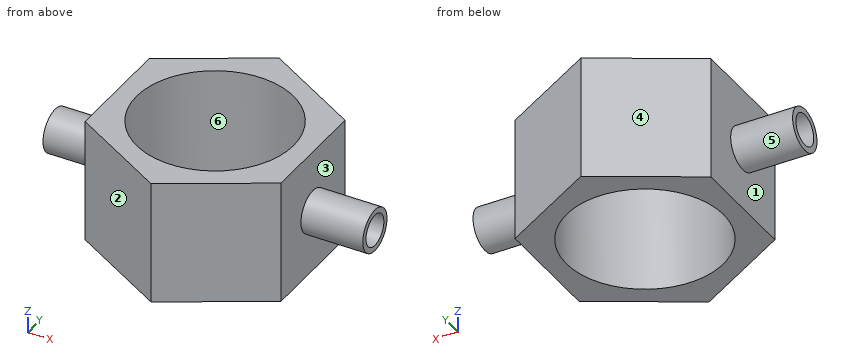
```python
from build123d import *

# Parameters (mm, degrees)
F1_DEPTH  = 12.7
F2_R      = 16.11687381
F3_DEPTH  = 25.4
F4_R      = 4.4261898193
F5_DEPTH  = 12.7
F6_R      = 4.3771900823
F7_DEPTH  = 12.7
F8_R      = 3.2385
F9_DEPTH  = 7.62
F10_R     = 3.2422174322
F11_DEPTH = 7.62


with BuildPart() as f1:
    # F0 (on Top) → F1 (new body, symmetric)
    with BuildSketch(Plane.XY):
        Polygon((-20.0972985476, -2.401636506), (-20.0972985476, -25.6079979589), (0, -37.2111786854), (20.0972985476, -25.6079979589), (20.0972985476, -2.401636506), (0, 9.2015442204), align=None)
    extrude(amount=F1_DEPTH, both=True)

    # F2 (on face) → F3 (cut)
    with BuildSketch(Plane.XY.offset(12.7)):
        with Locations((0, -14.0048172325)):
            Circle(F2_R)
    extrude(amount=-F3_DEPTH, mode=Mode.SUBTRACT)

    # F4 (on face) → F5 (join)
    with BuildSketch(Plane(origin=(-20.0972985476, 0, 0), x_dir=(0, -1, 0), z_dir=(-1, 0, 0))):
        with Locations((14.0048172325, 0)):
            Circle(F4_R)
    extrude(amount=F5_DEPTH)

    # F6 (on face) → F7 (join)
    with BuildSketch(Plane.YZ.offset(20.0972985476)):
        with Locations((-14.0048172325, 0)):
            Circle(F6_R)
    extrude(amount=F7_DEPTH)

    # F8 (on face) → F9 (cut)
    with BuildSketch(Plane(origin=(-32.7972985476, 0, 0), x_dir=(0, -1, 0), z_dir=(-1, 0, 0))):
        with Locations((14.0048172325, 0)):
            Circle(F8_R)
    extrude(amount=-F9_DEPTH, mode=Mode.SUBTRACT)

    # F10 (on face) → F11 (cut)
    with BuildSketch(Plane.YZ.offset(32.7972985476)):
        with Locations((-14.0048172325, 0)):
            Circle(F10_R)
    extrude(amount=-F11_DEPTH, mode=Mode.SUBTRACT)


solid = f1.part
```
Read the model definition and answer for the solid it produces. Units are mm, in the model's axes. Face numbers are marked on the shaded views. A direction names the side the tool comes from. Round coordinates to 2 decimals unless told otherwise and drop trailing zeros. Write each loop counter-clockwise with the first axis right and the second up, starting at its lowest first coordinate (ties: lowest second). Pieces come first, ordered by that corner, then holes. Notation, with made-up numbers: (9.25, -14) - (23.25, -14) arc R18 cw to (23.25, -7) - close; hole circle Ø1 at (-39.75, 88). An arc over 180 degrees is marked (long way). Use CSV: the item, a comma, the result in double quotes.
Q1. Find section A-A, the plane y = -5. Write down the section's boundary in (x, z).
Values:
outline,"(-20.1, -12.7) - (-13.37, -12.7) - (-13.37, 12.7) - (-20.1, 12.7) - close; (13.37, -12.7) - (20.1, -12.7) - (20.1, 12.7) - (13.37, 12.7) - close"
Q2. A tool of negligible diameter and unlimited length cuts with its end or side. For the marked faces 1, 2 and 3, from which of +Z, -Z, +X, -X, +Y, -Y can it reach the whole face along a straight path? Write none if from no direction.
Values:
face 1,"-X"
face 2,"+Z, -Z, -X, -Y"
face 3,"+X"
Q3. Find section D-D, the plane x = 24.5. Write down the section's boundary in (y, z).
Values:
outline,"circle Ø8.75 at (-14, 0)"
Q4. Each of these flat-tipped pins is pushed along its axis until it touches: pin 1 Ø4 at (x, z) = (-18.5, 4) entering from -Y; pin 2 Ø5 at (x, z) = (-12, 9) entering from -Y; pin 3 Ø1.9 at (y, z) = (-15, 1) entering from -X. Where does it stop, or does it pass through?
Values:
pin 1,"stops at y = -27.68"
pin 2,"stops at y = -31.73"
pin 3,"stops at x = -25.18"
Q5. Find section B-B, the plane x = -9. Write down the section's boundary in (y, z).
Values:
outline,"(-32.02, -12.7) - (-27.37, -12.7) - (-27.37, 12.7) - (-32.02, 12.7) - close; (-0.63, -12.7) - (4.01, -12.7) - (4.01, 12.7) - (-0.63, 12.7) - close"
Q6. Straight lines are drawn through the part: line 1 along Y through (x, z) = (0, -1.5); line 2 along X through (y, z) = (-16, -6); line 3 along X through (y, z) = (-28.5, -3.75). For each, find the intervals that lie inside material, in ascending order.
Values:
line 1,"y = -37.21 to -30.12, 2.11 to 9.2"
line 2,"x = -20.1 to -15.99, 15.99 to 20.1"
line 3,"x = -15.09 to -7.05, 7.05 to 15.09"
Q7. Find section C-C, the plane z = -11. Write down the section's boundary in (x, y).
Values:
outline,"(-20.1, -25.61) - (0, -37.21) - (20.1, -25.61) - (20.1, -2.4) - (0, 9.2) - (-20.1, -2.4) - close; hole circle Ø32.23 at (0, -14)"
Q8. Determine the mould class of the marked faces 4, 5 and 6 for opening direction Y: +Y half, -Y half, draft (parallel to the pull), parting line (faces both ways), or undercut.
Values:
face 4,"+Y half"
face 5,"parting line"
face 6,"undercut"
